from build123d import *

# Parameters (mm, degrees)
SKETCH013_W     = 44
SKETCH013_H     = 69
PAD006_DEPTH    = 1
SKETCH014_W     = 40
SKETCH014_H     = 64
SKETCH014_W_2   = 36
SKETCH014_H_2   = 60
PAD007_DEPTH    = 2
FILLET005_R     = 3
FILLET006_R     = 5
CHAMFER002_SIZE = 3
FILLET007_R     = 8
FILLET008_R     = 3
FILLET009_R     = 0.9
SKETCH015_W     = 2
SKETCH015_H     = 10
PAD008_DEPTH    = 6
FILLET011_R     = 2.5
SKETCH016_R     = 1
POCKET002_DEPTH = 41
SKETCH024_W     = 0.2
SKETCH024_H     = 50
POCKET007_DEPTH = 0.2


with BuildPart() as part:
    # Sketch013 → Pad006 (new body)
    with BuildSketch(Plane.XY):
        with Locations((0, 2.5)):
            Rectangle(SKETCH013_W, SKETCH013_H)
    extrude(amount=PAD006_DEPTH)

    # Sketch014 (on Face5 of Pad006) → Pad007 (join)
    with BuildSketch(Plane(origin=(0, 0, 0), x_dir=(1, 0, 0), z_dir=(0, 0, -1))):
        with Locations((0, -2)):
            Rectangle(SKETCH014_W, SKETCH014_H)
        with Locations((0, -2)):
            Rectangle(SKETCH014_W_2, SKETCH014_H_2, mode=Mode.SUBTRACT)
    extrude(amount=PAD007_DEPTH)

    # Fillet005
    fillet005_edges = [part.edges().sort_by_distance(p)[0] for p in [
        (18, 32, -1),
        (-18, 32, -1),
        (-18, -28, -1),
        (18, -28, -1),
    ]]
    fillet(fillet005_edges, radius=FILLET005_R)

    # Fillet006
    fillet006_edges = [part.edges().sort_by_distance(p)[0] for p in [
        (20, -30, -1),
        (-20, -30, -1),
        (-20, 34, -1),
        (20, 34, -1),
    ]]
    fillet(fillet006_edges, radius=FILLET006_R)

    # Chamfer002
    chamfer002_edges = [part.edges().sort_by_distance(p)[0] for p in [
        (22, 37, 0.5),
        (-22, 37, 0.5),
    ]]
    chamfer(chamfer002_edges, length=CHAMFER002_SIZE)

    # Fillet007
    fillet007_edges = [part.edges().sort_by_distance(p)[0] for p in [
        (-22, 34, 0.5),
        (22, 34, 0.5),
    ]]
    fillet(fillet007_edges, radius=FILLET007_R)

    # Fillet008
    fillet008_edges = [part.edges().sort_by_distance(p)[0] for p in [
        (-19, 37, 0.5),
        (19, 37, 0.5),
    ]]
    fillet(fillet008_edges, radius=FILLET008_R)

    # Fillet009
    fillet009_edges = [part.edges().sort_by_distance(p)[0] for p in [
        (-21.480851, 33.521227, 1),
        (-18.976175, 36.735386, 1),
        (-22, -0.656854, 1),
        (0, 37, 1),
        (0, -32, 1),
        (18.976175, 36.735386, 1),
        (22, -0.656854, 1),
        (21.480851, 33.521227, 1),
    ]]
    fillet(fillet009_edges, radius=FILLET009_R)

    # Sketch015 (on Face27 of Fillet009) → Pad008 (join)
    with BuildSketch(Plane(origin=(0, 0, -2), x_dir=(1, 0, 0), z_dir=(0, 0, -1))):
        with Locations((-19, 0)):
            Rectangle(SKETCH015_W, SKETCH015_H)
        with Locations((19, 0)):
            Rectangle(SKETCH015_W, SKETCH015_H)
    extrude(amount=PAD008_DEPTH)

    # Fillet011
    fillet011_edges = [part.edges().sort_by_distance(p)[0] for p in [
        (-19, -5, -2),
        (-19, -5, -8),
        (19, -5, -2),
        (19, -5, -8),
        (-19, 5, -8),
        (-19, 5, -2),
        (19, 5, -8),
        (19, 5, -2),
    ]]
    fillet(fillet011_edges, radius=FILLET011_R)

    # Sketch016 (on Face3 of Fillet011) → Pocket002 (cut)
    with BuildSketch(Plane(origin=(-20, 0, 0), x_dir=(0, -1, 0), z_dir=(-1, 0, 0))):
        with Locations((0, -5.5)):
            Circle(SKETCH016_R)
    extrude(amount=-POCKET002_DEPTH, mode=Mode.SUBTRACT)

    # Sketch024 (on Face57 of Pocket002) → Pocket007 (cut)
    with BuildSketch(Plane.XY.offset(1)):
        with Locations((0, 3)):
            Rectangle(SKETCH024_W, SKETCH024_H)
    extrude(amount=-POCKET007_DEPTH, mode=Mode.SUBTRACT)


with BuildPart() as part_1:
    # Body003 placement: moved
    add(part.part.moved(Location((0, -32, 52))))


solid = part_1.part
Geometry: final body of the model. Coordinates: model frame, mm. A direction names the side the tool comes from. Coordinates: 2 decimals unless noted, no trailing zeros. Order: outer loops, then holes, each group sorted by start corner. A loop starts at its lowest first (then second) coordinate and runs counter-clockwise, first axis right, second up. Notation, with made-up numbers: (13.25, 52.25) - (52.25, 52.25) arc R20 ccw to (52.25, 57.25) - close; hole circle Ø4 at (56, -28.5). An arc over 180 degrees is marked (long way). Use one line per item in the form item = value.
1) Ray query, L1, parallel to X at y = -30, z = 48; L2, parallel to Y at x = 4, z = 50.75; L3, parallel to Z at x = 19, y = -32. Return the intervals inside material, ascending.
Solutions:
L1 = -20 to -18, 18 to 20
L2 = -62 to -60, 0 to 2
L3 = 44 to 45.5, 47.5 to 53
2) Pin query (flat end, axial travel): pin 1 (8 mm diameter, centred on x = -9, y = -8, fed in from -Z); pin 2 (0.8 mm diameter, centred on x = -19.5, z = 47, fed in from -Y); pin 3 (5 mm diameter, centred on y = -53.5, z = 48.5, fed in from -X). Return the tip coordinate at first contact, or that it passes through.
Solutions:
pin_1 = 52
pin_2 = -37
pin_3 = -20
3) Mould query, pull axis Y, two halves, no side actions, for faces 6 (the face through (19.014, -36.287, 44.752)), 7 (the face through (0, -30, 52)), 8 (the face through (-19, -32, 44)). Classes: +Y half, -Y half, draft (parallel to the pull), parting line (faces both ways), or undercut.
Solutions:
face_6 = -Y half
face_7 = undercut
face_8 = draft
4) Set-up query: faces 1 (the face through (-19, -60, 51)), 2 (the face through (17.14, -59.1, 50.99)), 3 (the face through (-19, 0, 51)), 4 (the face through (20, -30, 50)), 5 (the face through (-0.1, 0.5, 50)). Return all of +Z, -Z, +X, -X, +Y, -Y with unobstructed straight access to the full face (end or side cutting, diameter ignored); none if empty.
Solutions:
face_1 = -Z, -X, -Y
face_2 = -Z
face_3 = -Z, -X, +Y
face_4 = -Z, +X, +Y, -Y
face_5 = -Z, +X, -X, +Y
5) Section A-A (y = -32). Return loops of the section in (x, z).
Solutions:
outline = (-22, 52) - (-20, 52) - (-20, 47.5) - (-18, 47.5) - (-18, 52) - (18, 52) - (18, 47.5) - (20, 47.5) - (20, 52) - (22, 52) - (22, 52.1) arc R0.9 ccw to (21.1, 53) - (0.1, 53) - (0.1, 52.8) - (-0.1, 52.8) - (-0.1, 53) - (-21.1, 53) arc R0.9 ccw to (-22, 52.1) - close; (-20, 44) - (-18, 44) - (-18, 45.5) - (-20, 45.5) - close; (18, 44) - (20, 44) - (20, 45.5) - (18, 45.5) - close
6) Section D-D (y = -9). Return loops of the section in (x, z).
Solutions:
outline = (-22, 52) - (-20, 52) - (-20, 50) - (-18, 50) - (-18, 52) - (18, 52) - (18, 50) - (20, 50) - (20, 52) - (22, 52) - (22, 52.1) arc R0.9 ccw to (21.1, 53) - (0.1, 53) - (0.1, 52.8) - (-0.1, 52.8) - (-0.1, 53) - (-21.1, 53) arc R0.9 ccw to (-22, 52.1) - close
7) Section B-B (z = 51). Return loops of the section in (x, y).
Solutions:
outline = (-20, -57) arc R5 ccw to (-15, -62) - (15, -62) arc R5 ccw to (20, -57) - (20, -3) arc R5 ccw to (15, 2) - (-15, 2) arc R5 ccw to (-20, -3) - close; hole (-18, -57) arc R3 ccw to (-15, -60) - (15, -60) arc R3 ccw to (18, -57) - (18, -3) arc R3 ccw to (15, 0) - (-15, 0) arc R3 ccw to (-18, -3) - close
8) Section C-C (x = -2). Return loops of the section in (y, z).
Solutions:
outline = (-64, 52) - (-62, 52) - (-62, 50) - (-60, 50) - (-60, 52) - (0, 52) - (0, 50) - (2, 50) - (2, 52) - (5, 52) - (5, 52.1) arc R0.9 ccw to (4.1, 53) - (-63.1, 53) arc R0.9 ccw to (-64, 52.1) - close
